The listing builds one solid part. Answer for the finished solid, in the listing's coordinates (mm). Round coordinates to 2 decimals unless told otherwise and drop trailing zeros. Write each loop counter-clockwise with the first axis right and the second up, starting at its lowest first coordinate (ties: lowest second). Pieces come first, ordered by that corner, then holes. Notation, with made-up numbers: (85, 44.25) - (89, 44.25) arc R24 cw to (89, 71.25) - close; hole circle Ø11 at (23, 60.5). An arc over 180 degrees is marked (long way). Return JSON: item names as keys, results as strings. Group by question number.
(1) Find the intervals of material crossed by line 1 along X through (y, z) = (-1.75, 0); line 2 along Y through (x, z) = (86.5, -64); line 3 along X through (y, z) = (-1.25, -30), in increasing order. Write a range as [from, to].
(2) Section A-A, the plane z = -24.5 is taken. Give the number of separate pieces and of enclosed holes in the cut face, then the cut area to 3 significant figures.
(3) Section C-C, the plane y = 12.5 is taken. Write down the section's boundary in (x, z), then the cut area to 3 significant figures.
(4) Section B-B, the plane x = 36.5 is taken. Write down the section's boundary in (y, z).
(5) Each of these flat-tipped pins is pushed along its axis until it touches: pin 1 (12 mm diameter, centred on x = -51.96, z = 30, fed in from -Y); pin 2 (13.5 mm diameter, centred on y = 20, z = 0, fed in from -X); pin 3 (8 mm diameter, centred on x = 60, z = -69, fed in from +Y); pin 4 (12 mm diameter, centred on x = -67.5, y = 0, fed in from -Z). Where does it stop, or does it pass through?
(6) Section D-D, the plane z = 76 is taken. Write down the section's boundary in (x, y), then the cut area to 3 significant figures.
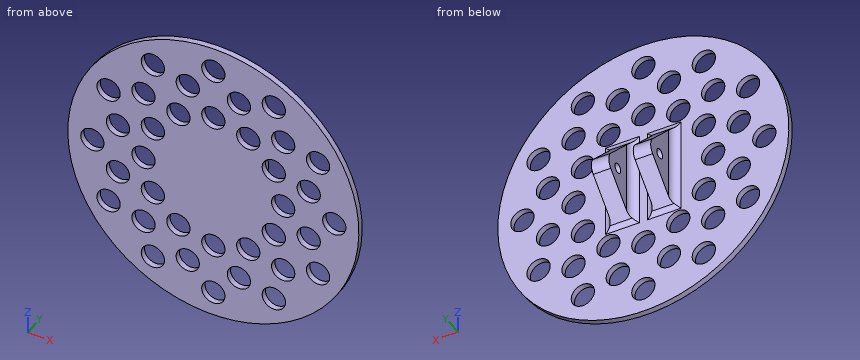
```python
from build123d import *

# Parameters (mm, degrees)
SKETCH1_R            = 125
BOSS_EXTRUDE1_DEPTH  = 5
SKETCH4_R            = 4.25
BOSS_EXTRUDE2_DEPTH  = 15
FILLET1_R            = 7
FILLET1_OF_MIRROR1_R = 7
SKETCH5_R            = 10
CUT_EXTRUDE1_DEPTH   = 15


with BuildPart() as part:
    # Sketch1 → Boss-Extrude1 (new body)
    with BuildSketch(Plane(origin=(0, 0, 0), x_dir=(1, 0, 0), z_dir=(0, 1, 0))):
        with Locations(Location((0, 0, 0), (0, 0, 270))):
            Circle(SKETCH1_R)
    extrude(amount=-BOSS_EXTRUDE1_DEPTH)

    # Sketch4 → Boss-Extrude2 (add)
    with BuildSketch(Plane(origin=(10.5, 0, 0), x_dir=(0, 0, -1), z_dir=(1, 0, 0))):
        with BuildLine():
            Line((37.67766953, 0), (-37.67766953, 0))
            Line((-37.67766953, 0), (-7.071067812, 30.606601718))
            ThreePointArc((-7.071067812, 30.606601718), (0, 33.535533906), (7.071067812, 30.606601718))
            Line((7.071067812, 30.606601718), (37.67766953, 0))
        make_face()
        with Locations((0, 20)):
            Circle(SKETCH4_R, mode=Mode.SUBTRACT)
    boss_extrude2 = extrude(amount=BOSS_EXTRUDE2_DEPTH)

    # Fillet1
    fillet1_edges = [part.edges().sort_by_distance(p)[0] for p in [
        (18, 0, 37.67766953),
        (18, 0, -37.67766953),
        (25.5, 0, 0),
        (10.5, 0, 0),
    ]]
    fillet(fillet1_edges, radius=FILLET1_R)

    # Mirror1: Boss-Extrude2 across plane
    add(boss_extrude2.mirror(Plane(origin=(0, 0, 0), x_dir=(0, 0, 1), z_dir=(1, 0, 0))))

    # Fillet1 of Mirror1
    fillet1_of_mirror1_edges = [part.edges().sort_by_distance(p)[0] for p in [
        (-18, 0, 37.67766953),
        (-18, 0, -37.67766953),
        (-25.5, 0, 0),
        (-10.5, 0, 0),
    ]]
    fillet(fillet1_of_mirror1_edges, radius=FILLET1_OF_MIRROR1_R)

    # Sketch5 → Cut-Extrude1 (cut)
    with BuildSketch(Plane(origin=(0, 0, 0), x_dir=(1, 0, 0), z_dir=(0, 1, 0))):
        with Locations(Location((-60, 0, 0), (0, 0, 270))):
            Circle(SKETCH5_R)
        with Locations(Location((-51.961524227, 30, 0), (0, 0, 270))):
            Circle(SKETCH5_R)
        with Locations(Location((-30, 51.961524227, 0), (0, 0, 270))):
            Circle(SKETCH5_R)
        with Locations(Location((0, 60, 0), (0, 0, 270))):
            Circle(SKETCH5_R)
        with Locations(Location((30, 51.961524227, 0), (0, 0, 270))):
            Circle(SKETCH5_R)
        with Locations(Location((51.961524227, 30, 0), (0, 0, 270))):
            Circle(SKETCH5_R)
        with Locations(Location((60, 0, 0), (0, 0, 270))):
            Circle(SKETCH5_R)
        with Locations(Location((51.961524227, -30, 0), (0, 0, 270))):
            Circle(SKETCH5_R)
        with Locations(Location((30, -51.961524227, 0), (0, 0, 270))):
            Circle(SKETCH5_R)
        with Locations(Location((0, -60, 0), (0, 0, 270))):
            Circle(SKETCH5_R)
        with Locations(Location((-30, -51.961524227, 0), (0, 0, 270))):
            Circle(SKETCH5_R)
        with Locations(Location((-51.961524227, -30, 0), (0, 0, 270))):
            Circle(SKETCH5_R)
        with Locations(Location((-81.961524227, 21.961524227, 0), (0, 0, 270))):
            Circle(SKETCH5_R)
        with Locations(Location((-60, 60, 0), (0, 0, 270))):
            Circle(SKETCH5_R)
        with Locations(Location((-21.961524227, 81.961524227, 0), (0, 0, 270))):
            Circle(SKETCH5_R)
        with Locations(Location((21.961524227, 81.961524227, 0), (0, 0, 270))):
            Circle(SKETCH5_R)
        with Locations(Location((60, 60, 0), (0, 0, 270))):
            Circle(SKETCH5_R)
        with Locations(Location((81.961524227, 21.961524227, 0), (0, 0, 270))):
            Circle(SKETCH5_R)
        with Locations(Location((81.961524227, -21.961524227, 0), (0, 0, 270))):
            Circle(SKETCH5_R)
        with Locations(Location((60, -60, 0), (0, 0, 270))):
            Circle(SKETCH5_R)
        with Locations(Location((21.961524227, -81.961524227, 0), (0, 0, 270))):
            Circle(SKETCH5_R)
        with Locations(Location((-21.961524227, -81.961524227, 0), (0, 0, 270))):
            Circle(SKETCH5_R)
        with Locations(Location((-60, -60, 0), (0, 0, 270))):
            Circle(SKETCH5_R)
        with Locations(Location((-81.961524227, -21.961524227, 0), (0, 0, 270))):
            Circle(SKETCH5_R)
        with Locations(Location((-103.923048454, 0, 0), (0, 0, 270))):
            Circle(SKETCH5_R)
        with Locations(Location((-90, 51.961524227, 0), (0, 0, 270))):
            Circle(SKETCH5_R)
        with Locations(Location((-51.961524227, 90, 0), (0, 0, 270))):
            Circle(SKETCH5_R)
        with Locations(Location((0, 103.923048454, 0), (0, 0, 270))):
            Circle(SKETCH5_R)
        with Locations(Location((51.961524227, 90, 0), (0, 0, 270))):
            Circle(SKETCH5_R)
        with Locations(Location((90, 51.961524227, 0), (0, 0, 270))):
            Circle(SKETCH5_R)
        with Locations(Location((103.923048454, 0, 0), (0, 0, 270))):
            Circle(SKETCH5_R)
        with Locations(Location((90, -51.961524227, 0), (0, 0, 270))):
            Circle(SKETCH5_R)
        with Locations(Location((51.961524227, -90, 0), (0, 0, 270))):
            Circle(SKETCH5_R)
        with Locations(Location((0, -103.923048454, 0), (0, 0, 270))):
            Circle(SKETCH5_R)
        with Locations(Location((-51.961524227, -90, 0), (0, 0, 270))):
            Circle(SKETCH5_R)
        with Locations(Location((-90, -51.961524227, 0), (0, 0, 270))):
            Circle(SKETCH5_R)
    extrude(amount=-CUT_EXTRUDE1_DEPTH, mode=Mode.SUBTRACT)


solid = part.part
```
Working result:
{
 "1": {"line 1": "x = [-125, -113.92], [-93.92, -70], [-50, 50], [70, 93.92], [113.92, 125]", "line 2": "y = [-5, 0]", "line 3": "x = [-121.35, -87.91], [-76.01, -61.96], [-41.96, 41.96], [61.96, 76.01], [87.91, 121.35]"},
 "2": {"separate pieces": "5", "enclosed holes": "0", "area": "1,300 mm^2"},
 "3": {"outline": "(-25.5, -25.18) - (-10.5, -25.18) - (-10.5, 25.18) - (-25.5, 25.18) - close; (10.5, -25.18) - (25.5, -25.18) - (25.5, 25.18) - (10.5, 25.18) - close", "area": "1,510 mm^2"},
 "4": {"outline": "(-5, -119.55) - (0, -119.55) - (0, -59.56) - (-5, -59.56) - close; (-5, -44.36) - (0, -44.36) - (0, 44.36) - (-5, 44.36) - close; (-5, 59.56) - (0, 59.56) - (0, 119.55) - (-5, 119.55) - close"},
 "5": {"pin 1": "passes through", "pin 2": "stops at x = -25.5", "pin 3": "stops at y = 0", "pin 4": "stops at z = -108.82"},
 "6": {"outline": "(-99.24, -5) - (-29.99, -5) - (-29.99, 0) - (-99.24, 0) - close; (-13.93, -5) - (13.93, -5) - (13.93, 0) - (-13.93, 0) - close; (29.99, -5) - (99.24, -5) - (99.24, 0) - (29.99, 0) - close", "area": "832 mm^2"}
}
